from build123d import *

# Parameters (mm, degrees)
BOSS_EXTRUDE1_DEPTH = 19.05
CUT_EXTRUDE1_DEPTH  = 10.795
FILLET1_R           = 0.3175
CHAMFER1_SIZE       = 0.3175


with BuildPart() as part:
    # Sketch1 → Boss-Extrude1 (new body)
    with BuildSketch(Plane(origin=(0, 0, 0), x_dir=(0, 0, -1), z_dir=(1, 0, 0))):
        with BuildLine():
            Line((3.4925, -2.286), (-3.4925, -2.286))
            Line((-3.4925, -2.286), (-4.133882072, -1.644617928))
            ThreePointArc((-4.133882072, -1.644617928), (-4.599127523, -0.948328904), (-4.7625, -0.127))
            Line((-4.7625, -0.127), (-4.7625, 0.127))
            ThreePointArc((-4.7625, 0.127), (-4.599127523, 0.948328904), (-4.133882072, 1.644617928))
            Line((-4.133882072, 1.644617928), (-3.4925, 2.286))
            Line((-3.4925, 2.286), (3.4925, 2.286))
            Line((3.4925, 2.286), (4.133882072, 1.644617928))
            ThreePointArc((4.133882072, 1.644617928), (4.599127523, 0.948328904), (4.7625, 0.127))
            Line((4.7625, 0.127), (4.7625, -0.127))
            ThreePointArc((4.7625, -0.127), (4.599127523, -0.948328904), (4.133882072, -1.644617928))
            Line((4.133882072, -1.644617928), (3.4925, -2.286))
        make_face()
    extrude(amount=BOSS_EXTRUDE1_DEPTH)

    # Sketch2 → Cut-Extrude1 (cut)
    with BuildSketch(Plane(origin=(19.05, 0, 0), x_dir=(0, 0, -1), z_dir=(1, 0, 0))):
        with BuildLine():
            ThreePointArc((-0.139499975, 0), (-1.051014863, 1.428430101), (-2.7305, 1.203482064))
            Line((-2.7305, 1.203482064), (-0.1905, -0.397553869))
            ThreePointArc((-0.1905, -0.397553869), (-0.15230201, -0.200405889), (-0.139499975, 0))
        make_face()
        with BuildLine():
            Line((-0.1905, -0.397553869), (-2.7305, 1.203482064))
            ThreePointArc((-2.7305, 1.203482064), (-2.554348209, -1.332396361), (-0.1905, -0.397553869))
        make_face()
        with BuildLine():
            Line((-2.7305, 2.286), (-2.7305, 1.203482064))
            ThreePointArc((-2.7305, 1.203482064), (-1.051014863, 1.428430101), (-0.139499975, 0))
            ThreePointArc((-0.139499975, 0), (-0.15230201, -0.200405889), (-0.1905, -0.397553869))
            Line((-0.1905, -0.397553869), (0.1905, -0.397553869))
            ThreePointArc((0.1905, -0.397553869), (0.874651791, 1.332396361), (2.7305, 1.203482064))
            Line((2.7305, 1.203482064), (2.7305, 2.286))
            Line((2.7305, 2.286), (-2.7305, 2.286))
        make_face()
        with BuildLine():
            ThreePointArc((2.7305, 1.203482064), (0.874651791, 1.332396361), (0.1905, -0.397553869))
            Line((0.1905, -0.397553869), (2.7305, 1.203482064))
        make_face()
        with BuildLine():
            Line((2.7305, 1.203482064), (0.1905, -0.397553869))
            ThreePointArc((0.1905, -0.397553869), (1.914905889, -1.56219799), (3.289500025, 0))
            ThreePointArc((3.289500025, 0), (3.142930101, 0.663485137), (2.7305, 1.203482064))
        make_face()
    extrude(amount=-CUT_EXTRUDE1_DEPTH, mode=Mode.SUBTRACT)

    # Fillet1
    fillet1_edges = [part.edges().sort_by_distance(p)[0] for p in [
        (13.6525, 2.286, 2.7305),
        (13.6525, 2.286, -2.7305),
    ]]
    fillet(fillet1_edges, radius=FILLET1_R)

    # Chamfer1
    chamfer1_edges = [part.edges().sort_by_distance(p)[0] for p in [
        (8.255, -0.397553869, 0),
    ]]
    chamfer(chamfer1_edges, length=CHAMFER1_SIZE)
    chamfer1_2_edges = [part.edges().sort_by_distance(p)[0] for p in [
        (8.255, 2.193006403, 2.823493597),
        (8.255, 1.585991032, 2.7305),
    ]]
    chamfer(chamfer1_2_edges, length=CHAMFER1_SIZE)
    chamfer1_3_edges = [part.edges().sort_by_distance(p)[0] for p in [
        (8.255, 1.585991032, -2.7305),
        (8.255, 2.193006403, -2.823493597),
    ]]
    chamfer(chamfer1_3_edges, length=CHAMFER1_SIZE)
    chamfer1_4_edges = [part.edges().sort_by_distance(p)[0] for p in [
        (8.255, -1.332396361, -2.554348209),
    ]]
    chamfer(chamfer1_4_edges, length=CHAMFER1_SIZE - 0.0001)  # a hair under: the kernel refuses the full size
    chamfer1_5_edges = [part.edges().sort_by_distance(p)[0] for p in [
        (8.255, -1.332396361, 2.554348209),
    ]]
    chamfer(chamfer1_5_edges, length=CHAMFER1_SIZE - 0.0001)  # a hair under: the kernel refuses the full size

    # Mirror1: part across plane


with BuildPart() as part_1:
    add(part.part)
    add(part.part.mirror(Plane(origin=(0, 0, 0), x_dir=(0, 0, 1), z_dir=(1, 0, 0))))


solid = part_1.part
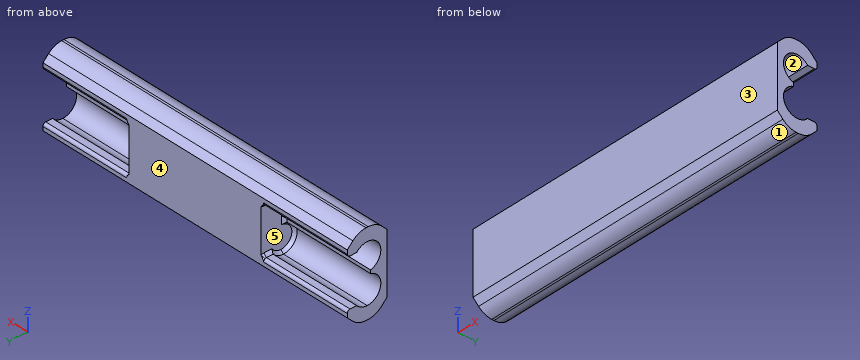
Geometry check sheet. Reference: the model listing, model coordinates, mm. Face numbers are marked on the shaded views. A direction names the side the tool comes from. Coordinates: 2 decimals unless noted, no trailing zeros. Order: outer loops, then holes, each group sorted by start corner. A loop starts at its lowest first (then second) coordinate and runs counter-clockwise, first axis right, second up. Notation, with made-up numbers: (-26.5, 57.5) -> (-7.5, 57.5) arc R18 ccw to (-7.5, 72.5) -> close; hole circle Ø8 at (-14, 76.5). An arc over 180 degrees is marked (long way). Use a Markdown table: item, result. Add a question column.
1. Mould release check, pull along Z, two halves, no side actions. Record for the marked faces 1, 2 and 3: pulls with the +Z half, pulls with the -Z half, needs draft (parallel to the pull), parting line crosses it, or undercut.
2. Go/stop test with flat-tipped pins: pin 1 Ø0.6 at (x, y) = (-12.5, 2) entering from +Z; pin 2 Ø0.6 at (x, y) = (12.5, 1.5) entering from +Z (3 decimals); pin 3 Ø1.5 at (x, y) = (6.5, 1) entering from +Z. Record where each tip stops, or that it passes through.
3. Cross-section at A-A (x = 2). Enter the section's corners in (y, z), and give its area (3 significant figures).
4. Set-up check for the marked faces 4 and 5: record each of +Z, -Z, +X, -X, +Y, -Y from which the full face is reachable in a straight line by a thin tool's end or side.
5. Material ranges on L1, parallel to Z at x = 14.5, y = 0; L2, parallel to Z at x = -13, y = -0.5; L3, parallel to X at y = 1.6, z = 1.25 (3 decimals), recorded low to high.
Filled sheet:
| question | item | result |
|---|---|---|
| 1 | face 1 | pulls with the -Z half |
| 1 | face 2 | undercut |
| 1 | face 3 | needs draft |
| 2 | pin 1 | z = 4.08 |
| 2 | pin 2 | z = 4.475 |
| 2 | pin 3 | z = 4.76 |
| 3 | outline | (-2.29, -3.49) -> (-1.64, -4.13) arc R2.15 ccw to (-0.13, -4.76) -> (0.13, -4.76) arc R2.15 ccw to (1.64, -4.13) -> (2.29, -3.49) -> (2.29, 3.49) -> (1.64, 4.13) arc R2.15 ccw to (0.13, 4.76) -> (-0.13, 4.76) arc R2.15 ccw to (-1.64, 4.13) -> (-2.29, 3.49) -> close |
| 3 | area | 39.9 mm2 |
| 4 | face 4 | +Z, -Z, +X, -X, +Y |
| 4 | face 5 | -X |
| 5 | L1 | -4.76 to -3.29, 3.29 to 4.76 |
| 5 | L2 | -4.73 to -3.21, -0.22 to 0.22, 3.21 to 4.73 |
| 5 | L3 | -8.255 to 8.255 |
